from build123d import *

# Parameters (mm, degrees)
PAD013_DEPTH = 14.7
FILLET007_R  = 0.3
BOX003_W     = 3.2
BOX003_H     = 16.6
BOX003_DEPTH = 1.6
FILLET011_R  = 1.59


with BuildPart() as part:
    # Sketch025 → Pad013 (new body)
    with BuildSketch(Plane.XY):
        with BuildLine():
            Line((-1.6, 0), (-6, 0))
            Line((-6, 0), (-6, 1.8))
            Line((-6, 1.8), (-0.9, 1.8))
            Line((-0.9, 1.8), (-0.9, 1.9))
            ThreePointArc((-0.9, 1.9), (-2.144796, 4.905204), (-5.15, 6.15))
            Line((-5.15, 6.15), (-6.8, 6.15))
            Line((-6.8, 6.15), (-6.8, 6.95))
            Line((-6.8, 6.95), (-5.15, 6.95))
            ThreePointArc((-0.1, 1.9), (-1.579111, 5.470889), (-5.15, 6.95))
            Line((-0.1, 1.8), (-0.1, 1.9))
            Line((0, 1.8), (-0.1, 1.8))
            Line((0, -1.8), (0, 1.8))
            Line((-1.6, -1.8), (0, -1.8))
            Line((-1.6, 0), (-1.6, -1.8))
        make_face()
    pad013 = extrude(amount=PAD013_DEPTH)

    # Mirrored005: Pad013 across Sketch025 V_Axis
    add(pad013.mirror(Plane(origin=(0, 0, 0), x_dir=(0, 0, 1), z_dir=(1, 0, 0))))

    # Fillet007
    fillet007_edges = [part.edges().sort_by_distance(p)[0] for p in [
        (6.8, 6.15, 7.35),
        (6.8, 6.95, 7.35),
        (-6.8, 6.95, 7.35),
        (-6.8, 6.15, 7.35),
    ]]
    fillet(fillet007_edges, radius=FILLET007_R)

    # Box003 → Box003 (join)
    with BuildSketch(Plane(origin=(-1.6, -1.8, 0), x_dir=(1, 0, 0), z_dir=(0, -1, 0))):
        with Locations((1.6, 8.3)):
            Rectangle(BOX003_W, BOX003_H)
    extrude(amount=BOX003_DEPTH)

    # Fillet011
    fillet011_edges = [part.edges().sort_by_distance(p)[0] for p in [
        (0, -3.4, 0),
    ]]
    fillet(fillet011_edges, radius=FILLET011_R)


with BuildPart() as part_1:
    # Body002 placement: moved
    add(part.part.moved(Location((-39, 1.8, 7.075))))


solid = part_1.part
The listing builds one solid part. Answer for the finished solid, in the listing's coordinates (mm). A direction names the side the tool comes from. Round coordinates to 2 decimals unless told otherwise and drop trailing zeros. Order: outer loops, then holes, each group sorted by start corner. A loop starts at its lowest first (then second) coordinate and runs counter-clockwise, first axis right, second up. Notation, with made-up numbers: (89, 30) -> (109, 30) arc R30 ccw to (109, 67) -> close; hole circle Ø9 at (73, 69.5). An arc over 180 degrees is marked (long way). Put each result on its own line as item: value.
Q1. Section B-B, the plane x = -42.25 is taken. Write down the section's boundary in (y, z) (3 decimals), and give its area (3 significant figures).
Results list:
outline: (1.8, 7.075) -> (3.6, 7.075) -> (3.6, 21.775) -> (1.8, 21.775) -> close; (7.502, 7.075) -> (8.379, 7.075) -> (8.379, 21.775) -> (7.502, 21.775) -> close
area: 39.4 mm^2
Q2. Which of the six approach directions +Z, -Z, +X, -X, +Y, -Y give full straight-line access (tool end or side, diameter ignored) to faces 1 (the flat face through (-40.6, 0, 15)), 2 (the flat face through (-39.5, 4.1, 21.775)), 3 (the cylindrical face through (-41.11, 6.67, 14.32)), 4 (the cylindrical face through (-36.89, 6.67, 14.32)), 5 (the flat face through (-35, 1.8, 14))?
Results list:
face 1: +Z, -Z, -X, -Y
face 2: +Z, +X, -X, +Y
face 3: +Z, -Z, -X
face 4: +Z, -Z, +X
face 5: +Z, -Z, +X, -Y
Q3. Each of these flat-tipped pins is pushed along its axis until it touches: P1, Ø1, axis at y = 6, z = 17.5, coming from the -X side; P2, Ø1, axis at x = -38.5, y = 5.5, coming from the +Z side (3 decimals); P3, Ø3.5, axis at x = -42, z = 13, coming from the -Y side; P4, Ø1.5, axis at y = 3, z = 19, coming from the +X side. Where does it stop, or does it pass through?
Results list:
P1: x = -40.95
P2: z = 21.775
P3: y = -1.6
P4: x = -33
Q4. Consider line 1 along Y through (x, z) = (-33.25, 21.5); line 2 along Z through (x, y) = (-35.25, 2.25) (3 decimals); line 3 along X through (y, z) = (3, 19.25). Determine where each line is inside the solid, lowest interval first.
Results list:
line 1: 1.8 to 3.6, 7.95 to 8.75
line 2: 7.075 to 21.775
line 3: -45 to -33
Q5. Section A-A, the plane y = 5.25 is taken. Write down the section's boundary in (x, z) (3 decimals).
Results list:
outline: (-40.193, 7.075) -> (-39.344, 7.075) -> (-39.344, 21.775) -> (-40.193, 21.775) -> close; (-38.656, 7.075) -> (-37.807, 7.075) -> (-37.807, 21.775) -> (-38.656, 21.775) -> close
Q6. Section D-D, the plane y = 0.25 is taken. Write down the section's boundary in (x, z) (3 decimals), and give its area (3 significant figures).
Results list:
outline: (-40.6, 7.075) -> (-37.4, 7.075) -> (-37.4, 21.775) -> (-40.6, 21.775) -> close
area: 47.0 mm^2
Q7. Section C-C, the plane z = 14 is taken. Write down the section's boundary in (x, y), and give its area (3 significant figures).
Results list:
outline: (-45.8, 8.25) arc R0.3 ccw to (-45.5, 7.95) -> (-44.15, 7.95) arc R4.25 cw to (-39.9, 3.7) -> (-39.9, 3.6) -> (-45, 3.6) -> (-45, 1.8) -> (-40.6, 1.8) -> (-40.6, -1.6) -> (-37.4, -1.6) -> (-37.4, 1.8) -> (-33, 1.8) -> (-33, 3.6) -> (-38.1, 3.6) -> (-38.1, 3.7) arc R4.25 cw to (-33.85, 7.95) -> (-32.5, 7.95) arc R0.3 ccw to (-32.2, 8.25) -> (-32.2, 8.45) arc R0.3 ccw to (-32.5, 8.75) -> (-33.85, 8.75) arc R5.05 ccw to (-38.9, 3.7) -> (-38.9, 3.6) -> (-39.1, 3.6) -> (-39.1, 3.7) arc R5.05 ccw to (-44.15, 8.75) -> (-45.5, 8.75) arc R0.3 ccw to (-45.8, 8.45) -> close
area: 46.9 mm^2
Q8. Determine the mould class of faces 6 (the flat face through (-45, 7.95, 14)), 7 (the flat face through (-43, 1.8, 14)), 8 (the flat face through (-33, 8.75, 14)), 9 (the flat face through (-42, 3.6, 14)) for opening direction Y: pulls with the +Y half, pulls with the -Y half, needs draft (parallel to the pull), parting line crosses it, or undercut.
Results list:
face 6: undercut
face 7: pulls with the -Y half
face 8: pulls with the +Y half
face 9: undercut
